```python
from build123d import *

# Parameters (mm, degrees)
SKETCH1_W               = 47
SKETCH1_H               = 54
BOSS_EXTRUDE1_DEPTH     = 2
SKETCH2_W               = 6
SKETCH2_H               = 6
BOSS_EXTRUDE2_DEPTH     = 15
CHAMFER1_SIZE           = 5.3
CHAMFER2_SIZE           = 8.3
SKETCH3_R               = 1.5
CUT_EXTRUDE1_DEPTH      = 50.733694815
CHAMFER3_SIZE           = 2.8
CHAMFER4_SIZE           = 2
SKETCH4_W               = 6
SKETCH4_H               = 2
BOSS_EXTRUDE3_DEPTH     = 26.8
SKETCH6_W               = 6
SKETCH6_H               = 6
BOSS_EXTRUDE4_DEPTH     = 22
CHAMFER5_SIZE           = 8.1
CUT_EXTRUDE2_DEPTH      = 61.457423035
CHAMFER6_SIZE           = 8.1
CUT_EXTRUDE3_DEPTH      = 53.832588428
CUT_EXTRUDE3_DEPTH_BACK = 53.832588428
SKETCH8_R               = 1.5


with BuildPart() as part:
    # Sketch1 → Boss-Extrude1 (new body)
    with BuildSketch(Plane(origin=(0, 0, 0), x_dir=(1, 0, 0), z_dir=(0, 1, 0))):
        Rectangle(SKETCH1_W, SKETCH1_H)
    extrude(amount=BOSS_EXTRUDE1_DEPTH)

    # Sketch2 → Boss-Extrude2 (add)
    with BuildSketch(Plane.XZ):
        with Locations((-12.48, 24)):
            Rectangle(SKETCH2_W, SKETCH2_H)
        with Locations((20.5, 24)):
            Rectangle(SKETCH2_W, SKETCH2_H)
        with Locations((20.5, -24)):
            Rectangle(SKETCH2_W, SKETCH2_H)
        with Locations((-12.48, -24)):
            Rectangle(SKETCH2_W, SKETCH2_H)
    extrude(amount=BOSS_EXTRUDE2_DEPTH)

    # Chamfer1
    chamfer1_edges = [part.edges().sort_by_distance(p)[0] for p in [
        (-15.48, -15, 24),
        (-15.48, -15, -24),
    ]]
    chamfer(chamfer1_edges, length=CHAMFER1_SIZE)

    # Chamfer2
    # the kernel refuses this chamfer: 8.3 mm, written as the material it takes off along each edge
    with BuildSketch(Plane(origin=(23.5, -15, 0.3449688), x_dir=(0.027495876610586414, 0.9996219169112966, 0), z_dir=(0, 0, -1)), Plane(origin=(23.5, -15, -0.3449688), x_dir=(-0.9996219169112969, -0.027495876610586417, 0), z_dir=(0, 0, 1))) as chamfer2_piece_1:
        Polygon((CHAMFER2_SIZE * 0.999621916911, -CHAMFER2_SIZE * 0.0274958766106), (-CHAMFER2_SIZE * 0.0274958766106, -CHAMFER2_SIZE * 0.999621916911), (0, 0), align=None)
    extrude(amount=48.6899376, mode=Mode.SUBTRACT)

    # Sketch3 → Cut-Extrude1 (cut, through all)
    with BuildSketch(Plane.ZY.offset(15.48)):
        with Locations((24.5, -5)):
            Circle(SKETCH3_R)
        with Locations((-24.5, -5)):
            Circle(SKETCH3_R)
        with Locations((24.5, -15)):
            Circle(SKETCH3_R)
        with Locations((-24.5, -15)):
            Circle(SKETCH3_R)
    extrude(amount=-CUT_EXTRUDE1_DEPTH, mode=Mode.SUBTRACT)

    # Chamfer3
    chamfer3_edges = [part.edges().sort_by_distance(p)[0] for p in [
        (-15.48, 0, 24),
        (-15.48, 0, -24),
    ]]
    chamfer(chamfer3_edges, length=CHAMFER3_SIZE)

    # Chamfer4
    chamfer4_edges = [part.edges().sort_by_distance(p)[0] for p in [
        (-9.48, 0, 24),
        (-9.48, 0, -24),
    ]]
    chamfer(chamfer4_edges, length=CHAMFER4_SIZE)

    # Sketch4 → Boss-Extrude3 (add)
    with BuildSketch(Plane.ZY.offset(23.5)):
        with Locations((24, 1)):
            Rectangle(SKETCH4_W, SKETCH4_H)
        with Locations((-24, 1)):
            Rectangle(SKETCH4_W, SKETCH4_H)
    extrude(amount=BOSS_EXTRUDE3_DEPTH)

    # Sketch6 → Boss-Extrude4 (add)
    with BuildSketch(Plane.XZ):
        with Locations((-47.3, 24)):
            Rectangle(SKETCH6_W, SKETCH6_H)
        with Locations((-47.3, -24)):
            Rectangle(SKETCH6_W, SKETCH6_H)
    extrude(amount=BOSS_EXTRUDE4_DEPTH)

    # Chamfer5
    # the kernel refuses this chamfer: 8.1 mm, written as the material it adds along each edge
    with BuildSketch(Plane(origin=(-23.5, 2, 21), x_dir=(0.027495876610586174, 0, -0.9996219169112968), z_dir=(0, -1, 0)), Plane(origin=(-23.5, 2, -21), x_dir=(-0.9996219169112968, 0, -0.02749587661058618), z_dir=(0, -1, 0))) as chamfer5_piece_1:
        Polygon((CHAMFER5_SIZE * 0.999621916911, -CHAMFER5_SIZE * 0.0274958766106), (-CHAMFER5_SIZE * 0.0274958766106, -CHAMFER5_SIZE * 0.999621916911), (0, 0), align=None)
    extrude(amount=2)
    with BuildSketch(Plane(origin=(-44.3, 0, 27), x_dir=(-0.027495876610586608, -0.9996219169112968, 0), z_dir=(0, 0, -1))) as chamfer5_piece_2:
        Polygon((CHAMFER5_SIZE * 0.999621916911, -CHAMFER5_SIZE * 0.0274958766106), (-CHAMFER5_SIZE * 0.0274958766106, -CHAMFER5_SIZE * 0.999621916911), (0, 0), align=None)
    extrude(amount=6)
    with BuildSketch(Plane(origin=(-44.3, 0, -27), x_dir=(-0.027495876610586608, -0.9996219169112968, 0), z_dir=(0, 0, 1))) as chamfer5_piece_3:
        Polygon((CHAMFER5_SIZE * 0.999621916911, CHAMFER5_SIZE * 0.0274958766106), (-CHAMFER5_SIZE * 0.0274958766106, CHAMFER5_SIZE * 0.999621916911), (0, 0), align=None)
    extrude(amount=6)
    # the kernel refuses this chamfer: 8.1 mm, written as the material it takes off along each edge
    with BuildSketch(Plane(origin=(-50.3, -22, 0.169367797), x_dir=(0.9996219169112968, -0.027495876610586167, 0), z_dir=(0, 0, 1)), Plane(origin=(-50.3, -22, -0.169367797), x_dir=(-0.027495876610586608, 0.9996219169112968, 0), z_dir=(0, 0, -1))) as chamfer5_2_piece_1:
        Polygon((CHAMFER5_SIZE * 0.999621916911, CHAMFER5_SIZE * 0.0274958766106), (-CHAMFER5_SIZE * 0.0274958766106, CHAMFER5_SIZE * 0.999621916911), (0, 0), align=None)
    extrude(amount=47.661264405, mode=Mode.SUBTRACT)

    # Sketch7 → Cut-Extrude2 (cut, through all)
    with BuildSketch(Plane.XZ):
        Polygon((9.4, 21), (17.5, 21), (23.5, 21), (23.5, -21), (17.5, -21), (9.4, -21), (4.8, -21), (-3.3, -12.9), (-3.3, 12.9), (4.8, 21), align=None)
    extrude(amount=-CUT_EXTRUDE2_DEPTH, mode=Mode.SUBTRACT)

    # Chamfer6
    # the kernel refuses this chamfer: 8.1 mm, written as the material it adds along each edge
    with BuildSketch(Plane(origin=(17.5, 0, 27), x_dir=(0.02749587661058618, -0.9996219169112968, 0), z_dir=(0, 0, -1))) as chamfer6_piece_1_section:
        Polygon((CHAMFER6_SIZE * 0.999621916911, CHAMFER6_SIZE * 0.0274958766106), (-CHAMFER6_SIZE * 0.0274958766106, CHAMFER6_SIZE * 0.999621916911), (0, 0), align=None)
    chamfer6_piece_1 = extrude(amount=6, mode=Mode.PRIVATE)
    chamfer6_piece_1 = chamfer6_piece_1 - Plane(origin=(14.692276243, -5, 24.5), x_dir=(0, 0, 1), z_dir=(-1, 0, 0)) * Cylinder(1.5, 45, mode=Mode.PRIVATE)
    add(chamfer6_piece_1)
    with BuildSketch(Plane(origin=(17.5, 0, -27), x_dir=(0.02749587661058618, -0.9996219169112968, 0), z_dir=(0, 0, 1))) as chamfer6_piece_2_section:
        Polygon((CHAMFER6_SIZE * 0.999621916911, -CHAMFER6_SIZE * 0.0274958766106), (-CHAMFER6_SIZE * 0.0274958766106, -CHAMFER6_SIZE * 0.999621916911), (0, 0), align=None)
    chamfer6_piece_2 = extrude(amount=6, mode=Mode.PRIVATE)
    chamfer6_piece_2 = chamfer6_piece_2 - Plane(origin=(14.692276222, -5, -24.5), x_dir=(0, 0, 1), z_dir=(-1, 0, 0)) * Cylinder(1.5, 45, mode=Mode.PRIVATE)
    add(chamfer6_piece_2)

    # Sketch8 → Cut-Extrude3 (cut, two sides: drawn at the far end of the back side and taken through both)
    with BuildSketch(Plane(origin=(-9.48, 0, 0), x_dir=(0, 0, -1), z_dir=(1, 0, 0)).offset(-CUT_EXTRUDE3_DEPTH_BACK)):
        with Locations(Location((-24.5, -5, 0), (0, 0, 180))):
            Circle(SKETCH8_R)
        with Locations(Location((24.5, -5, 0), (0, 0, 180))):
            Circle(SKETCH8_R)
    extrude(amount=CUT_EXTRUDE3_DEPTH + CUT_EXTRUDE3_DEPTH_BACK, mode=Mode.SUBTRACT)


solid = part.part
```
Build history of the part. All positions in model axes, mm. A direction names the side the tool comes from. Round coordinates to 2 decimals unless told otherwise and drop trailing zeros. Order: outer loops, then holes, each group sorted by start corner. A loop starts at its lowest first (then second) coordinate and runs counter-clockwise, first axis right, second up. Notation, with made-up numbers: (38.25, -40) -> (85.25, -40) arc R18 ccw to (85.25, -24) -> close; hole circle Ø6 at (-8, 22.5). An arc over 180 degrees is marked (long way). Answer in a Markdown table with one row per item.
1) Band-saw the part on B-B on z = 24.5. Give the number of separate pieces and of enclosed holes in the cut face, and give its area (3 significant figures).
Values:
| item | result |
|---|---|
| separate pieces | 4 |
| enclosed holes | 0 |
| area | 380 mm2 |
2) Band-saw the part on A-A on y = -11.75. Give the cut face in (x, z), and give its area (3 significant figures).
Values:
| item | result |
|---|---|
| outline | (-50.3, -27) -> (-44.3, -27) -> (-44.3, -21) -> (-50.3, -21) -> close; (-50.3, 21) -> (-44.3, 21) -> (-44.3, 27) -> (-50.3, 27) -> close; (-13.43, -27) -> (-9.48, -27) -> (-9.48, -21) -> (-13.43, -21) -> close; (-13.43, 21) -> (-9.48, 21) -> (-9.48, 27) -> (-13.43, 27) -> close; (17.5, -27) -> (18.45, -27) -> (18.45, -21) -> (17.5, -21) -> close; (17.5, 21) -> (18.45, 21) -> (18.45, 27) -> (17.5, 27) -> close |
| area | 131 mm2 |
3) Which spindle directions (+Z, -Z, +X, -X, +Y, -Y) get a long thin tool onto all of the face, cutting with end or side? Do faces 1 (the flat face through (-13, 0, 0)), 2 (the flat face through (16, -2, -21)), 3 (the flat face through (-23.5, 1, 0)), 4 (the cylindrical face through (-10.4, -13.5, -24.5)), 5 (the flat face through (-9.48, -8, 24)). Say none if no direction does.
Values:
| item | result |
|---|---|
| face 1 | -Y |
| face 2 | +X, +Y, -Y |
| face 3 | -X, +Y, -Y |
| face 4 | +X, -Y |
| face 5 | +Z, -Z, -Y |
4) Band-saw the part on C-C on x = -17. Give the cut face in (y, z).
Values:
| item | result |
|---|---|
| outline | (-1.28, -27) -> (2, -27) -> (2, 27) -> (-1.28, 27) -> (-1.28, 21) -> (0, 21) -> (0, -21) -> (-1.28, -21) -> close |
5) Wall check: L1, parallel to Z at x = -42.75, y = -5; L2, parallel to Y at x = -13.65, z = 24.5; L3, parallel to Y at x = -47.5, z = -24.5. Give the ranges that are in metal, low to high.
Values:
| item | result |
|---|---|
| L1 | -27 to -26, -23 to -21, 21 to 23, 26 to 27 |
| L2 | -11.53 to -6.5, -3.5 to 2 |
| L3 | -16.7 to -6.5, -3.5 to 2 |
6) Mould opens along Y. For faces 6 (the flat face through (-8.47, -0.99, -24.04)), 7 (the flat face through (-44.3, -14, -24)), 8 (the cylindrical face through (-46.238, -3.536, 24.175)) say: released by +Y, released by -Y, zero draft, split by the parting line, or undercut.
Values:
| item | result |
|---|---|
| face 6 | released by -Y |
| face 7 | zero draft |
| face 8 | undercut |
7) Pin check, flat tips, straight feed: P1, Ø5, axis at y = -14, z = 23, coming from the +X side; P2, Ø1.5, axis at x = -8, y = -15.5, coming from the +Z side; P3, Ø0.8, axis at x = -10, z = -26.5, coming from the -Y side; P4, Ø1, axis at y = 1, z = -2, coming from the -X side. Stop position of each tip, or through.
Values:
| item | result |
|---|---|
| P1 | x = 18.7 |
| P2 | through |
| P3 | y = -15 |
| P4 | x = -23.5 |
